```python
from build123d import *

# Parameters (mm, degrees)
F2_DEPTH = 100
F3_DEPTH = 76
F4_DEPTH = 70
F5_DEPTH = 6
F7_DEPTH = 12.5


with BuildPart() as f2:
    # F0 (on Front) → F2 (new body)
    with BuildSketch(Plane.XZ):
        Polygon((-6.2, 0), (0, 0), (6.2, 0), (15, 0), (15, 7), (8.8388347648, 7), (0, 7), (-8.8388347648, 7), (-15, 7), (-15, 0), align=None)
        Polygon((0, -2.7), (0, 0), (-6.2, 0), (-8.9, -2.7), align=None)
        Polygon((6.2, 0), (0, 0), (0, -2.7), (8.9, -2.7), align=None)
    extrude(amount=-F2_DEPTH)

    # F1 (on Front) → F3 (join)
    with BuildSketch(Plane.XZ):
        with BuildLine():
            ThreePointArc((0, 7), (-12.9945857106, 19.6248437535), (-0.75, 32.9783473524))
            Line((-0.75, 32.9783473524), (-0.75, 44.9783473524))
            Line((-0.75, 44.9783473524), (-3.75, 44.9783473524))
            Line((-3.75, 44.9783473524), (-3.75, 36.5812393988))
            ThreePointArc((-3.75, 36.5812393988), (-16.3309227117, 24.7223895842), (-12.0208152802, 7.9791847198))
            Line((-12.0208152802, 7.9791847198), (-12.0208152802, 7))
            Line((-12.0208152802, 7), (0, 7))
        make_face()
        with BuildLine():
            ThreePointArc((0.75, 32.9783473524), (12.9945857106, 19.6248437535), (0, 7))
            Line((0, 7), (12.0208152802, 7))
            Line((12.0208152802, 7), (12.0208152802, 7.9791847198))
            ThreePointArc((12.0208152802, 7.9791847198), (16.3309227117, 24.7223895842), (3.75, 36.5812393988))
            Line((3.75, 36.5812393988), (3.75, 44.9783473524))
            Line((3.75, 44.9783473524), (0.75, 44.9783473524))
            Line((0.75, 44.9783473524), (0.75, 32.9783473524))
        make_face()
    extrude(amount=-F3_DEPTH)

    # F1 (on Front) → F4 (cut)
    with BuildSketch(Plane.XZ):
        with BuildLine():
            ThreePointArc((0, 7), (-12.9945857106, 19.6248437535), (-0.75, 32.9783473524))
            Line((-0.75, 32.9783473524), (-0.75, 44.9783473524))
            Line((-0.75, 44.9783473524), (-3.75, 44.9783473524))
            Line((-3.75, 44.9783473524), (-3.75, 36.5812393988))
            ThreePointArc((-3.75, 36.5812393988), (-16.3309227117, 24.7223895842), (-12.0208152802, 7.9791847198))
            Line((-12.0208152802, 7.9791847198), (-12.0208152802, 7))
            Line((-12.0208152802, 7), (0, 7))
        make_face()
        with BuildLine():
            ThreePointArc((0.75, 32.9783473524), (12.9945857106, 19.6248437535), (0, 7))
            Line((0, 7), (12.0208152802, 7))
            Line((12.0208152802, 7), (12.0208152802, 7.9791847198))
            ThreePointArc((12.0208152802, 7.9791847198), (16.3309227117, 24.7223895842), (3.75, 36.5812393988))
            Line((3.75, 36.5812393988), (3.75, 44.9783473524))
            Line((3.75, 44.9783473524), (0.75, 44.9783473524))
            Line((0.75, 44.9783473524), (0.75, 32.9783473524))
        make_face()
    extrude(amount=-F4_DEPTH, mode=Mode.SUBTRACT)

    # F0 (on Front) → F5 (join)
    with BuildSketch(Plane.XZ):
        with BuildLine():
            Line((-8.8388347648, 11.1611652352), (-8.8388347648, 7))
            Line((-8.8388347648, 7), (0, 7))
            Line((0, 7), (0, 11.5))
            ThreePointArc((0, 11.5), (-8.4907228952, 19.602980205), (-0.7931729561, 28.4629118311))
            Line((-0.7931729561, 28.4629118311), (-0.7931729561, 40.4629118311))
            Line((-0.7931729561, 40.4629118311), (-3.624006873, 40.4629118311))
            Line((-3.624006873, 40.4629118311), (-3.624006873, 31.9631339617))
            ThreePointArc((-3.624006873, 31.9631339617), (-12.1248126232, 23.0395589899), (-8.8388347648, 11.1611652352))
        make_face()
        with BuildLine():
            Line((0, 7), (8.8388347648, 7))
            Line((8.8388347648, 7), (8.8388347648, 11.1611652352))
            ThreePointArc((8.8388347648, 11.1611652352), (12.1248126232, 23.0395589899), (3.624006873, 31.9631339617))
            Line((3.624006873, 31.9631339617), (3.624006873, 40.4629118311))
            Line((3.624006873, 40.4629118311), (0.7931729561, 40.4629118311))
            Line((0.7931729561, 40.4629118311), (0.7931729561, 28.4629118311))
            ThreePointArc((0.7931729561, 28.4629118311), (8.4907228952, 19.602980205), (0, 11.5))
            Line((0, 11.5), (0, 7))
        make_face()
    extrude(amount=-F5_DEPTH)

    # F6 (on Right) → F7 (cut, symmetric)
    with BuildSketch(Plane.YZ):
        with BuildLine():
            ThreePointArc((73, 60.07835), (71.5, 58.57835), (73, 57.07835))
            Line((73, 57.07835), (73, 58.57835))
            Line((73, 58.57835), (73, 60.07835))
        make_face()
        with BuildLine():
            Line((73, 58.57835), (73, 57.07835))
            ThreePointArc((73, 57.07835), (74.0606601718, 57.5176898282), (74.5, 58.57835))
            ThreePointArc((74.5, 58.57835), (74.0606601718, 59.6390101718), (73, 60.07835))
            Line((73, 60.07835), (73, 58.57835))
        make_face()
        with BuildLine():
            ThreePointArc((4.5, 54.06291), (4.0606601718, 55.1235701718), (3, 55.56291))
            ThreePointArc((3, 55.56291), (1.9393398282, 53.0022498282), (4.5, 54.06291))
        make_face()
    extrude(amount=F7_DEPTH, both=True, mode=Mode.SUBTRACT)


solid = f2.part
```
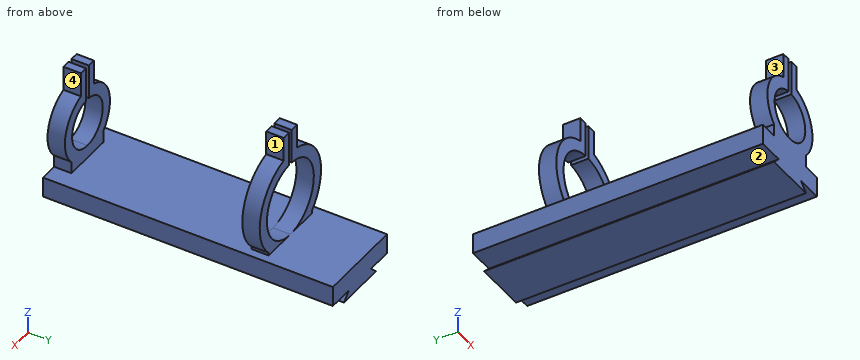
The model under review builds one solid part; all positions refer to its coordinate system, in mm. Face numbers are marked on the shaded views. A direction names the side the tool comes from. Give positions to 0.01 mm unless a question says otherwise; leave off trailing zeros. Write each loop counter-clockwise with the first axis right and the second up, starting at its lowest first coordinate (ties: lowest second). Pieces come first, ordered by that corner, then holes.
(1) Consider section C-C, the plane y = 78.5. Give the boundary of the cut face in (x, z).
(2) To check wall thickness, follow L1, parallel to Y at x = -10, z = 17; L2, parallel to Z at x = -13, y = 8; L3, parallel to Z at x = -1, y = 50. State the ranges of each line that lie inside material, in increasing order.
(3) Tool access review of the marked faces 1, 2, 3 and 4: name each direction out of +Z, -Z, +X, -X, +Y, -Y from which nothing blocks a thin tool from reaching the whole face with its end or side.
(4) For P1, Ø3, axis at y = 72.5, z = 39, coming from the -X side; P2, Ø1.8, axis at y = 2, z = 34.5, coming from the -X side; P3, Ø18.5, axis at x = -11.5, z = 23.5, coming from the -Y side; P4, Ø5, axis at y = 74.5, z = 40, coming from the +X side, all flat-tipped, find the tip position at first contact; note any pin that passes through.
(5) Consider section D-D, the plane z = 20. Give the boundary of the cut face in (x, y).
(6) Consider section A-A, the plane z = 39. Give the boundary of the cut face in (x, y), and give its area (3 significant figures).
(7) Consider section B-B, the plane x = -10. Give the boundary of the cut face in (y, z).
Returned:
1. outline: (-15, 0) - (-6.2, 0) - (-8.9, -2.7) - (8.9, -2.7) - (6.2, 0) - (15, 0) - (15, 7) - (-15, 7) - close
2. L1: y = 0 to 6
2. L2: z = 0 to 7
2. L3: z = -2.7 to 7
3. face 1: +Z, +X, +Y, -Y
3. face 2: -X, +Y, -Y
3. face 3: +Z, -X, -Y
3. face 4: +Z, +X, -Y
4. P1: stops at x = -3.75
4. P2: stops at x = -3.62
4. P3: stops at y = 0
4. P4: stops at x = 3.75
5. outline: (-17, 70) - (-13, 70) - (-13, 76) - (-17, 76) - close; (-12.5, 0) - (-8.5, 0) - (-8.5, 6) - (-12.5, 6) - close; (8.5, 0) - (12.5, 0) - (12.5, 6) - (8.5, 6) - close; (13, 70) - (17, 70) - (17, 76) - (13, 76) - close
6. outline: (-3.75, 70) - (-0.75, 70) - (-0.75, 76) - (-3.75, 76) - close; (-3.62, 0) - (-0.79, 0) - (-0.79, 6) - (-3.62, 6) - close; (0.75, 70) - (3.75, 70) - (3.75, 76) - (0.75, 76) - close; (0.79, 0) - (3.62, 0) - (3.62, 6) - (0.79, 6) - close
6. area: 70.0 mm2
7. outline: (0, 0) - (100, 0) - (100, 7) - (76, 7) - (76, 11.69) - (70, 11.69) - (70, 7) - (0, 7) - close; (0, 12.5) - (6, 12.5) - (6, 27.5) - (0, 27.5) - close; (70, 28.31) - (76, 28.31) - (76, 33.75) - (70, 33.75) - close
